Source: three-view drawing plus pictorial views. Frame: mm from the lowest corner of the part. Give positions to 0.01 mm unless a question says otherwise; leave off trailing zeros. Write each loop counter-clockwise with the first axis right and the second up, starting at its lowest first coordinate (ties: lowest second). Pieces come first, ordered by that corner, then holes. Notation, with made-up numbers: (26.25, 51) -> (72.25, 51) arc R29 cw to (72.25, 90) -> close; hole circle Ø1 at (1, 45). An arc over 180 degrees is marked (long way). Answer in a Markdown table with one row per item. Add a question column.
Item 1: Section query B-B on y = 4.25. Output: boundary loops of the cut face in (x, z) (1 decimal).
Item 2: Draft query along Z for the marked faces 1, 2 and 3. Return one class per face: +Z half, -Z half, draft (parallel to the pull), parting line (faces both ways), or undercut.
Item 3: Section query A-A on x = 12.7. Output: boundary loops of the cut face in (y, z) (1 decimal).
Item 4: Section query D-D on x = 21.5. Output: boundary loops of the cut face in (y, z), plus the area to 3 significant figures.
Item 5: Material intervals for probe 1 along Z at (x, y) = (12.5, 5); probe 2 along Z at (x, y) = (7.75, 9.75); probe 3 along X at (y, z) = (15.5, 59.5) (1 decimal), sorted ascending. Write a range as from..to.
Item 6: Section query C-C on z = 17. Output: boundary loops of the cut face in (x, y).
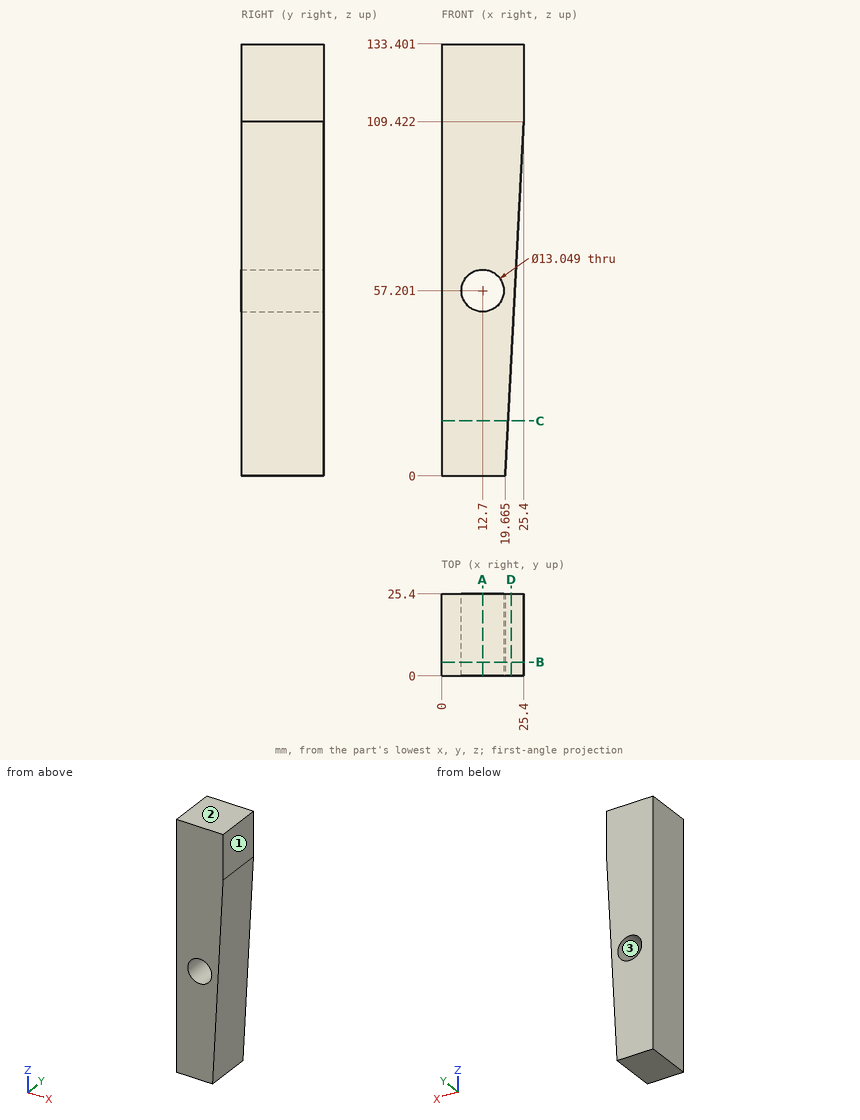
Findings below:
| question | item | result |
|---|---|---|
| 1 | outline | (0, 0) -> (19.7, 0) -> (25.4, 109.4) -> (25.4, 133.4) -> (0, 133.4) -> close; hole circle Ø13 at (12.7, 57.2) |
| 2 | face 1 | draft |
| 2 | face 2 | +Z half |
| 2 | face 3 | undercut |
| 3 | outline | (0, 0) -> (25.4, 0) -> (25.4, 50.7) -> (0, 50.7) -> close; (0, 63.7) -> (25.4, 63.7) -> (25.4, 133.4) -> (0, 133.4) -> close |
| 4 | outline | (0, 35.01) -> (25.4, 35.01) -> (25.4, 133.4) -> (0, 133.4) -> close |
| 4 | area | 2,500 mm^2 |
| 5 | probe 1 | z = 0..50.68, 63.72..133.4 |
| 5 | probe 2 | z = 0..52.95, 61.45..133.4 |
| 5 | probe 3 | x = 0..6.6, 18.8..22.8 |
| 6 | outline | (0, 0) -> (20.56, 0) -> (20.56, 25.4) -> (0, 25.4) -> close |
